Here's how the part is built. I have some questions about the finished solid (model axes, mm). Face numbers are marked on the shaded views. Round coordinates to 2 decimals unless told otherwise and drop trailing zeros. Order: outer loops, then holes, each group sorted by start corner. A loop starts at its lowest first (then second) coordinate and runs counter-clockwise, first axis right, second up. Notation, with made-up numbers: (67.5, -11.5) -> (109.5, -11.5) arc R29 ccw to (109.5, 14.5) -> close; hole circle Ø11 at (76, 86.5). An arc over 180 degrees is marked (long way). Use a Markdown table: item, result. Add a question column.
(1) I'm going to push flat-ended pins straight in: P1, Ø5, axis at x = 84, y = 41.5, coming from the -Z side; P2, Ø6, axis at x = 144, z = 209.5, coming from the +Y side; P3, Ø2, axis at x = -159, z = 491.5, coming from the -Y side. Where does each tip first touch, or does it pass through?
(2) I want a section at A-A, the plane x = 0. Please give me the cut outline in (y, z).
(3) If I drill on probe 1 along Y at (x, z) = (0, 282); probe 2 along Y at (x, z) = (5, 500); probe 3 along Z at (x, y) = (-42.5, 68.5), over which ranges is the centre line in solid material (lowest first)?
(4) I want a section at C-C, the plane z = 270.5. Please give me the cut outline in (x, y), then the cut area to 3 significant figures.
(5) Thinking about a two-plate mould opening in Y: for the marked faces 1, 2 and 3, which applies, pulls with the +Y half, pulls with the -Y half, needs draft (parallel to the pull), parting line crosses it, or undercut?
from build123d import *

# Parameters (mm, degrees)
F0_R      = 216.727836
F1_DEPTH  = 116.332
F1_FACE_R = 216.727836
F3_DEPTH  = 520.7
F2_R      = 190.087444
F4_DEPTH  = 594.36


with BuildPart() as f1:
    # F0 (on Top) → F1 (new body)
    with BuildSketch(Plane.XY):
        Circle(F0_R)
    extrude(amount=F1_DEPTH)

    # F1_face (on face) → F3 (join)
    with BuildSketch(Plane.XY.offset(116.332)):
        Circle(F1_FACE_R)
    extrude(amount=F3_DEPTH)

    # F2 (on Top) → F4 (cut)
    with BuildSketch(Plane.XY):
        Circle(F2_R)
    extrude(amount=F4_DEPTH, mode=Mode.SUBTRACT)


solid = f1.part
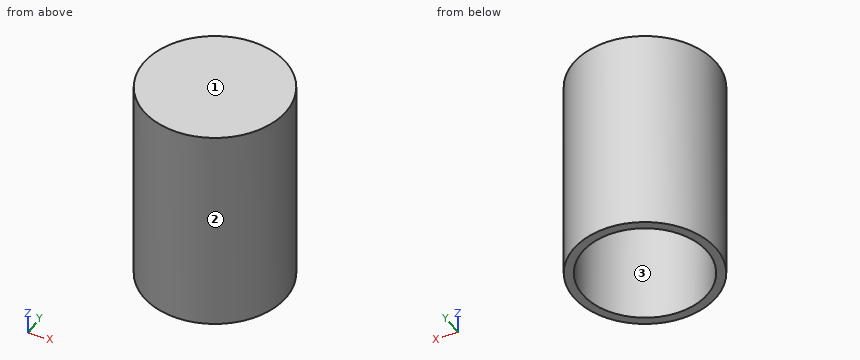
Taken from the geometry:
| question | item | result |
|---|---|---|
| 1 | P1 | stops at z = 594.36 |
| 1 | P2 | stops at y = 164.59 |
| 1 | P3 | stops at y = -148.35 |
| 2 | outline | (-216.73, 0) -> (-190.09, 0) -> (-190.09, 594.36) -> (190.09, 594.36) -> (190.09, 0) -> (216.73, 0) -> (216.73, 637.03) -> (-216.73, 637.03) -> close |
| 3 | probe 1 | y = -216.73 to -190.09, 190.09 to 216.73 |
| 3 | probe 2 | y = -216.67 to -190.02, 190.02 to 216.67 |
| 3 | probe 3 | z = 594.36 to 637.03 |
| 4 | outline | circle Ø433.46 at (0, 0); hole circle Ø380.17 at (0, 0) |
| 4 | area | 34,000 mm2 |
| 5 | face 1 | needs draft |
| 5 | face 2 | parting line crosses it |
| 5 | face 3 | undercut |
